from build123d import *

# Parameters (mm, degrees)
F0_W     = 498
F0_H     = 130
F1_DEPTH = 449
F2_T     = -2


with BuildPart() as f1:
    # F0 (on Top) → F1 (new body)
    with BuildSketch(Plane.XY):
        with Locations((249, 65)):
            Rectangle(F0_W, F0_H)
    extrude(amount=-F1_DEPTH)

    # F2
    f2_openings = [f1.faces().sort_by_distance(p)[0] for p in [
        (249, 0, -224.5),
        (249, 65, 0),
    ]]
    offset(amount=F2_T, openings=f2_openings)


solid = f1.part
For this review, take the finished solid that the model builds, in its own axes (mm). A direction names the side the tool comes from. Round coordinates to 2 decimals unless told otherwise and drop trailing zeros. Loops run counter-clockwise (first coordinate to the right, second up) from the corner with the lowest first, then second, coordinate; pieces in that order, holes last. Notation, with made-up numbers: (-17, 55.25) - (4, 55.25) arc R25 ccw to (4, 82.25) - close; hole circle Ø3 at (11, 14.25). An arc over 180 degrees is marked (long way). One line per item, written item: value. Start each with the question number.
Item 1: For L1, parallel to X at y = 69, z = -111.5; L2, parallel to Z at x = 407, y = 8; L3, parallel to Y at x = 385, z = -91, list the stretches that pass through material, from the lowest coordinate up.
Item 2: Clearance check with flat-ended pins moving along their axes: pin 1 Ø2 at (x, y) = (171.5, 49) entering from +Z; pin 2 Ø6 at (x, z) = (164, -45.5) entering from -Y. State where each tip first meets the part, or that it passes through.
Item 3: Take a section at B-B (z = -270). Give the boundary of the cut face in (x, y).
Item 4: Take a section at C-C (x = 101). Give the boundary of the cut face in (y, z).
Item 5: For faces 1 (the flat face through (496, 63, -220)), 2 (the flat face through (498, 64, -221)), list the 3-axis set-ups (+Z, -Z, +X, -X, +Y, -Y) from which the entire face can be reached by the end or side of a thin tool; tool diameter is ignored.
Item 6: Take a section at A-A (y = 73). Give the boundary of the cut face in (x, z), plus the area to 3 significant figures.
Item 7: The part is to be moulded in two halves that separate along X. For faces 3 (the flat face through (0, 64, -221)), 4 (the flat face through (2, 63, -220)), 5 (the flat face through (246, 66, -449)), say which applies: +X half, -X half, draft (parallel to the pull), parting line (faces both ways), or undercut.
Answer below:
1. L1: x = 0 to 2, 496 to 498
1. L2: z = -449 to -447
1. L3: y = 128 to 130
2. pin 1: stops at z = -447
2. pin 2: stops at y = 128
3. outline: (0, 0) - (2, 0) - (2, 128) - (496, 128) - (496, 0) - (498, 0) - (498, 130) - (0, 130) - close
4. outline: (0, -449) - (130, -449) - (130, 0) - (128, 0) - (128, -447) - (0, -447) - close
5. face 1: +Z, -Y
5. face 2: +Z, -Z, +X, +Y, -Y
6. outline: (0, -449) - (498, -449) - (498, 0) - (496, 0) - (496, -447) - (2, -447) - (2, 0) - (0, 0) - close
6. area: 2,780 mm2
7. face 3: -X half
7. face 4: undercut
7. face 5: draft
